For this review, take the finished solid that the model builds, in its own axes (mm). Face numbers are marked on the shaded views. A direction names the side the tool comes from. Coordinates: 2 decimals unless noted, no trailing zeros. Write each loop counter-clockwise with the first axis right and the second up, starting at its lowest first coordinate (ties: lowest second). Pieces come first, ordered by that corner, then holes. Notation, with made-up numbers: M 79.5,13 L 120.5,13 A20 cw 120.5,50 Z; hole C 87.5,51.25 d1. An arc over 180 degrees is marked long. Return JSON: item names as keys, results as strings.
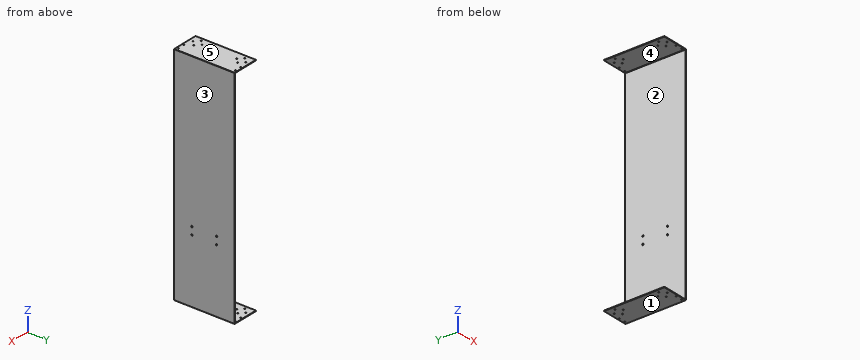
Autodesk Inventor part; units mm, degrees
ref_plane "YZ Plane" through (0, 0, 0) normal (1, 0, 0) x (0, 1, 0)
ref_plane "XZ Plane" through (0, 0, 0) normal (0, 1, 0) x (-1, 0, 0)
ref_plane "XY Plane" through (0, 0, 0) normal (0, 0, 1) x (1, 0, 0)
sketch "Sketch1" plane through (0, 0, 0) normal (0, 1, 0) x (-1, 0, 0)
  line L0 (1, 0) -> (70.5, 0)
  line L1 (0, -1) -> (0, -593)
  line L2 (1, -594) -> (70.5, -594)
  line L3 (70.5, -1.6) -> (2.6, -1.6)
  line L4 (1.6, -2.6) -> (1.6, -591.4)
  line L5 (2.6, -592.4) -> (70.5, -592.4)
  line L6 (70.5, 0) -> (70.5, -1.6)
  line L7 (70.5, -592.4) -> (70.5, -594)
  arc A0 (1, 0) -> (0, -1) centre (1, -1) ccw
  arc A1 (0, -593) -> (1, -594) centre (1, -593) ccw
  arc A2 (2.6, -1.6) -> (1.6, -2.6) centre (2.6, -2.6) ccw
  arc A3 (1.6, -591.4) -> (2.6, -592.4) centre (2.6, -591.4) ccw
  point P0 (0, 0)
  point P1 (0, -594)
  dimension "d0" = 70.5
  dimension "d1" = 594
  dimension "d2" = 70.5
  dimension "d3" = 1.6
  dimension "d4" = 1
  dimension "d5" = 1
extrude "Extrusion1" add sketch "Sketch1" along normal mid plane 160
sketch "Sketch2" plane through (-70.5, -80, 0) normal (0, 0, 1) x (1, 0, 0)
  line L0 (0, 0) -> (0, 160)
  line L1 (67.9, 160) -> (0, 160)
  line L2 (0, 0) -> (67.9, 0)
  circle A0 centre (20.9, 10) radius 1.75
  circle A1 centre (8.9, 22) radius 1.75
  circle A2 centre (20.9, 34) radius 1.75
  circle A3 centre (32.9, 22) radius 1.75
  line L3 (70.5, 80) -> (70.5, 160)
hole "Hole1" at (-49.6, -70, 0) at (-37.6, -58, 0) at (-49.6, -46, 0) at (-61.6, -58, 0) direction (0, 0, -1) diameter 3 end through all
mirror "Mirror1" about plane through (0, 0, 0) normal (0, 1, 0) of "Hole1"
sketch "Sketch3" plane through (-1.6, -80, -2.6) normal (-1, 0, 0) x (0, 0, 1)
  line L0 (-589.8, 0) -> (-589.8, 160)
  line L1 (-588.8, 160) -> (0, 160)
  line L2 (0, 0) -> (-588.8, 0)
  line L3 (-588.8, 0) -> (-588.8, 160)
  circle A0 centre (-420.4, 112.5) radius 2
  circle A1 centre (-400.4, 112.5) radius 2
  point P0 (2.6, 80)
  dimension "d28" = 4
  dimension "d30" = 4
  dimension "d33" = 47.5
  dimension "d35" = 20
extrude "Extrusion2" cut sketch "Sketch3" against normal blind 3
mirror "Mirror2" about plane through (0, 0, 0) normal (0, 1, 0) of "Extrusion2"
sketch "Sketch4" plane through (-1, 80, -594) normal (0, 0, -1) x (-1, 0, 0)
  line L0 (69.5, 0) -> (1.6, 0)
  line L1 (1.6, 0) -> (8.6, 0)
  circle A0 centre (7.61, -4.6) radius 2
  circle A1 centre (25.61, -4.6) radius 2
  line L2 (0, -160) -> (0, 0)
  line L3 (69.5, -160) -> (69.5, 0)
  point P0 (-1, -80)
  dimension "d38" = 4
  dimension "d40" = 4
  dimension "d48" = 4.6
  dimension "d49" = 4.6
  dimension "d51" = 18
  dimension "d52" = 43.89
hole "Hole2" at (-26.61, 75.4, -594) at (-8.61, 75.4, -594) direction (0, 0, 1) diameter 3 end through all
mirror "Mirror3" about plane through (0, 0, 0) normal (0, 1, 0) of "Hole2"
properties part number "Caja - Base"
1. Clearance check with a flat-ended pin moving along its axis: pin 1 Ø5 at (y, z) = (-32.5, -403) entering from -X. State where the tip first meets the part, or that it passes through.
Checks:
{"pin 1": "x = -1.6"}
2. Draft analysis for pull direction Z (two halves, no side actions). For the marked faces 1, 2 and 3, state which applies: +Z half, -Z half, draft (parallel to the pull), parting line (faces both ways), or undercut.
Checks:
{"face 1": "-Z half", "face 2": "undercut", "face 3": "draft"}
3. Wall thickness on L1, parallel to Y at x = -37.6, z = -0.7; L2, parallel to Y at x = -8.61, z = -593.1; L3, parallel to Z at x = -49.5, y = 35.5: over which ranges is each line inside the solid? List them lowest first. Write a range as from..to.
Checks:
{"L1": "-80..-59.5, -56.5..56.5, 59.5..80", "L2": "-80..-76.9, -73.9..73.9, 76.9..80", "L3": "-594..-592.4, -1.6..0"}
4. For the marked faces 4 and 5, list the 3-axis set-ups (+Z, -Z, +X, -X, +Y, -Y) from which the entire face can be reached by the end or side of a thin tool; tool diameter is ignored.
Checks:
{"face 4": "-X, +Y, -Y", "face 5": "+Z, +X, -X, +Y, -Y"}
5. We need section B-B (z = -491). State the section outline as (x, y) points.
Checks:
{"outline": "M -1.6,-80 L 0,-80 L 0,80 L -1.6,80 Z"}
6. We need section A-A (y = 8). State the section outline as (x, z) points, plus the area to 3 significant figures.
Checks:
{"outline": "M -70.5,-594 L -1,-594 A1 ccw 0,-593 L 0,-1 A1 ccw -1,0 L -70.5,0 L -70.5,-1.6 L -2.6,-1.6 A1 cw -1.6,-2.6 L -1.6,-591.4 A1 cw -2.6,-592.4 L -70.5,-592.4 Z", "area": "1,170 mm2"}
